Source: CAD feature listing. Evaluate the final solid. Frame: model axes, mm. A direction names the side the tool comes from. Give positions to 0.01 mm unless a question says otherwise; leave off trailing zeros. Answer in a Markdown table with one row per item.
Autodesk Inventor part; units mm, degrees
ref_plane "YZ Plane" through (0, 0, 0) normal (1, 0, 0) x (0, 1, 0)
ref_plane "XZ Plane" through (0, 0, 0) normal (0, 1, 0) x (-1, 0, 0)
ref_plane "XY Plane" through (0, 0, 0) normal (0, 0, 1) x (1, 0, 0)
sketch "Sketch1" plane through (0, 0, 0) normal (0, 0, 1) x (1, 0, 0)
  circle A0 centre (0, 12.7) radius 3.175
  circle A1 centre (-0.0751, 0) radius 3.175
  line L0 (-0.0751, 0) -> (-0.0751, 19.0499)
  line L1 (-0.0751, 3.175) -> (-0.0751, 24.8386)
  line L2 (6.35, 15.5543) -> (6.35, 5.2605)
  line L3 (9.525, 2.0855) -> (15.8376, 2.0855)
  line L4 (-6.5001, 15.5229) -> (-6.5001, 5.2772)
  line L5 (-9.6751, 2.1022) -> (-15.8387, 2.1022)
  arc A2 (-19.0064, -1.2874) -> (19.0051, -1.3074) centre (0, 0) ccw
  arc A3 (3.81, 18.6651) -> (-3.9901, 18.6274) centre (0, 0) ccw
  arc A4 (-3.9901, 18.6274) -> (-6.5001, 15.5229) centre (-3.3251, 15.5229) ccw
  arc A5 (6.35, 15.5543) -> (3.81, 18.6651) centre (3.175, 15.5543) ccw
  arc A6 (6.35, 5.2605) -> (9.525, 2.0855) centre (9.525, 5.2605) ccw
  arc A7 (-9.6751, 2.1022) -> (-6.5001, 5.2772) centre (-9.6751, 5.2772) ccw
  arc A8 (-15.8387, 2.1022) -> (-19.0064, -1.2874) centre (-15.8387, -1.0728) ccw
  arc A9 (19.0051, -1.3074) -> (15.8376, 2.0855) centre (15.8376, -1.0895) ccw
  point P0 (6.35, 17.9605)
  point P1 (6.35, 2.0855)
  point P2 (18.9355, 2.0855)
  point P3 (-6.5001, 2.1022)
  point P4 (-18.9337, 2.1022)
  point P5 (-6.5001, 17.9067)
  dimension "d6" = 6.35
  dimension "d3" = 6.35
  dimension "d11" = 15.875
  dimension "d12" = 3.175
extrude "Extrusion1" add sketch "Sketch1" along normal blind 12.7 contours A0 L0 | L0 A0 | A1 | L2 A6 L3 A9 A2 A8 L5 A7 L4 A4 A3 A5
draft "FaceDraft1" angle 2.5 pull direction (0, 0, 1) faces at (6.35, 8.6918, 4.2333) (4.713, 18.3319, 8.4667) (6.5695, 4.1006, 8.4667) (2.9511, 18.82, 4.2333) (13.7334, 2.0855, 4.2333) (-6.0664, 17.1247, 8.4667) (16.3313, 2.0469, 8.4667) (-6.5001, 12.1076, 4.2333) (18.5791, -4.2093, 8.4667) (-7.8866, 2.6539, 8.4667) (-16.0862, 2.0925, 4.2333) (-11.7296, 2.1022, 4.2333) fixed edges at (6.35, 10.4074, 12.7) (5.6343, 17.5623, 12.7) (7.2799, 3.0154, 12.7) (-0.092, 19.0498, 12.7) (12.6813, 2.0855, 12.7) (-5.7941, 17.519, 12.7) (18.1584, 1.0772, 12.7) (-6.5001, 10.4, 12.7) (-0.01, -19.05, 12.7) (-7.43, 3.0321, 12.7) (-18.1584, 1.0951, 12.7) (-12.7569, 2.1022, 12.7)
properties part number "Crank Cast Image"
(1) Ray query, probe 1 along X at (y, z) = (-11, 7.25); probe 2 along X at (y, z) = (-8, 11.5); probe 3 along Y at (x, z) = (6.5, 3). Return the intervals inside material, ascending.
A:
| item | result |
|---|---|
| probe 1 | x = -15.84 to 15.84 |
| probe 2 | x = -17.35 to 17.35 |
| probe 3 | y = -18.36 to 16.93 |
(2) Access query for faces 1 (the flat face through (-12.714, 2.383, 6.261)), 2 (the flat face through (6.63, 10.48, 6.26)), 3 (the flat face through (0, -4, 0)). Directions: +Z, -Z, +X, -X, +Y, -Y. A direction counts if a zero-diameter tool reaches every point of the face in a straight line with its end or side. Return the directions, or none.
A:
| item | result |
|---|---|
| face 1 | +Z, -X, +Y |
| face 2 | +Z, +X, +Y |
| face 3 | -Z, +X, -X, +Y, -Y |
(3) First-contact query: pin 1 Ø3 at (x, z) = (6.5, 9.5) entering from +Y; pin 2 Ø1 at (x, y) = (-14.5, -14) entering from +Z; pin 3 Ø1 at (x, z) = (9.5, 6.5) entering from +Y; pin 4 Ø4 at (y, z) = (0.5, 8.5) entering from -X. Flat tips, straight axial feed; report the tip coordinate or a pass-through.
A:
| item | result |
|---|---|
| pin 1 | stops at y = 18.32 |
| pin 2 | passes through |
| pin 3 | stops at y = 2.41 |
| pin 4 | stops at x = -19.26 |
